```python
from build123d import *

# Parameters (mm, degrees)
F1_DEPTH = 27.813
F3_DEPTH = 6.3119
F5_DEPTH = 4.699
F7_DEPTH = 5.08


with BuildPart() as f1:
    # F0 (on Top) → F1 (new body)
    with BuildSketch(Plane.XY):
        with BuildLine():
            Line((-18.8019596104, 10.1706712406), (-18.8019596104, -14.8356287594))
            Line((-18.8019596104, -14.8356287594), (-12.4900596104, -14.8356287594))
            Line((-12.4900596104, -14.8356287594), (-12.4900596104, -1.8752787594))
            ThreePointArc((-12.4900596104, -1.8752787594), (-6.4067596104, 4.2080212406), (-0.3234596104, -1.8752787594))
            Line((-0.3234596104, -1.8752787594), (-0.3234596104, -14.8356287594))
            Line((-0.3234596104, -14.8356287594), (5.9884403896, -14.8356287594))
            Line((5.9884403896, -14.8356287594), (5.9884403896, 10.1706712406))
            Line((5.9884403896, 10.1706712406), (-18.8019596104, 10.1706712406))
        make_face()
    extrude(amount=F1_DEPTH)

    # F2 (on face) → F3 (cut, through all)
    with BuildSketch(Plane.YZ.offset(5.9884403896)):
        with BuildLine():
            ThreePointArc((-7.9141287594, 21.6408), (-8.4869693167, 23.0237594426), (-9.8699287594, 23.5966))
            Line((-9.8699287594, 23.5966), (-9.8699287594, 21.6408))
            Line((-9.8699287594, 21.6408), (-9.8699287594, 19.685))
            ThreePointArc((-9.8699287594, 19.685), (-8.4869693167, 20.2578405574), (-7.9141287594, 21.6408))
        make_face()
        with BuildLine():
            Line((-9.8699287594, 21.6408), (-9.8699287594, 23.5966))
            ThreePointArc((-9.8699287594, 23.5966), (-11.252888202, 23.0237594426), (-11.8257287594, 21.6408))
            Line((-11.8257287594, 21.6408), (-9.8699287594, 21.6408))
        make_face()
        with BuildLine():
            Line((-9.8699287594, 19.685), (-9.8699287594, 21.6408))
            Line((-9.8699287594, 21.6408), (-11.8257287594, 21.6408))
            ThreePointArc((-11.8257287594, 21.6408), (-11.252888202, 20.2578405574), (-9.8699287594, 19.685))
        make_face()
        with BuildLine():
            ThreePointArc((-7.8475873364, 5.3523653187), (-8.4441574212, 6.7586539368), (-9.8699287594, 7.3070330344))
            Line((-9.8699287594, 7.3070330344), (-9.8699287594, 5.4864))
            Line((-9.8699287594, 5.4864), (-9.8699287594, 3.3976976029))
            ThreePointArc((-9.8699287594, 3.3976976029), (-8.4441574212, 3.9460767006), (-7.8475873364, 5.3523653187))
        make_face()
        with BuildLine():
            Line((-9.8699287594, 5.4864), (-9.8699287594, 7.3070330344))
            ThreePointArc((-9.8699287594, 7.3070330344), (-11.1622464384, 6.7590122471), (-11.7545891057, 5.4864))
            Line((-11.7545891057, 5.4864), (-9.8699287594, 5.4864))
        make_face()
        with BuildLine():
            ThreePointArc((-11.7545891057, 5.4864), (-11.2554518403, 4.0421507116), (-9.8699287594, 3.3976976029))
            Line((-9.8699287594, 3.3976976029), (-9.8699287594, 5.4864))
            Line((-9.8699287594, 5.4864), (-11.7545891057, 5.4864))
        make_face()
    extrude(amount=-F3_DEPTH, mode=Mode.SUBTRACT)

    # F4 (on face) → F5 (join)
    with BuildSketch(Plane(origin=(0, 10.1706712406, 0), x_dir=(-1, 0, 0), z_dir=(0, 1, 0))):
        with BuildLine():
            ThreePointArc((-3.9818403896, 14.5669), (-1.9582997195, 9.6816406701), (2.9269596104, 7.6581))
            Line((2.9269596104, 7.6581), (2.9269596104, 13.34135))
            ThreePointArc((2.9269596104, 13.34135), (2.0603648947, 13.7003052843), (1.7014096104, 14.5669))
            Line((1.7014096104, 14.5669), (-3.9818403896, 14.5669))
        make_face()
        with BuildLine():
            Line((2.9269596104, 13.34135), (2.9269596104, 7.6581))
            ThreePointArc((2.9269596104, 7.6581), (7.8122189403, 9.6816406701), (9.8357596104, 14.5669))
            ThreePointArc((9.8357596104, 14.5669), (2.9269596104, 21.4757), (-3.9818403896, 14.5669))
            Line((-3.9818403896, 14.5669), (1.7014096104, 14.5669))
            ThreePointArc((1.7014096104, 14.5669), (2.0603648947, 15.4334947157), (2.9269596104, 15.79245))
            ThreePointArc((2.9269596104, 15.79245), (3.7935543261, 15.4334947157), (4.1525096104, 14.5669))
            ThreePointArc((4.1525096104, 14.5669), (3.7935543261, 13.7003052843), (2.9269596104, 13.34135))
        make_face()
    extrude(amount=F5_DEPTH)

    # F6 (on face) → F7 (cut)
    with BuildSketch(Plane(origin=(0, 10.1706712406, 0), x_dir=(-1, 0, 0), z_dir=(0, 1, 0))):
        with BuildLine():
            Line((3.5874825428, 23.4577979645), (6.1019596104, 27.813))
            Line((6.1019596104, 27.813), (-5.9884403896, 27.813))
            Line((-5.9884403896, 27.813), (-5.9884403896, 14.4474878907))
            Line((-5.9884403896, 14.4474878907), (-5.9881597655, 14.637636653))
            ThreePointArc((-5.9881597655, 14.637636653), (-3.11318956, 21.1244113541), (3.5874825428, 23.4577979645))
        make_face()
    extrude(amount=-F7_DEPTH, mode=Mode.SUBTRACT)


solid = f1.part
```
Work out the finished part from the listing and answer in its coordinate system (mm). A direction names the side the tool comes from. Round coordinates to 2 decimals unless told otherwise and drop trailing zeros. Loops run counter-clockwise (first coordinate to the right, second up) from the corner with the lowest first, then second, coordinate; pieces in that order, holes last. Notation, with made-up numbers: M 63.5,2.25 L 106.5,2.25 A10 cw 106.5,14.25 Z; hole C -29.5,33 d3. An arc over 180 degrees is marked long. One line per question, with ' | ' between items.
Q1. A tool of negligible diameter and unlimited length cuts with its end or side. For faces 1 (the flat face through (-12.49, -8, 14)), 2 (the flat face through (-12, 1, 27.813)), 3 (the flat face through (-3, 10.171, 15)), from which of +Z, -Z, +X, -X, +Y, -Y can it reach the whole face along a straight path? Write none if from no direction.
Conclusion:
face 1: +Z, -Z, -Y | face 2: +Z, +X, -X, +Y, -Y | face 3: +Y
Q2. Consider line 1 along X through (y, z) = (-3, 24.25); line 2 along Y through (x, z) = (4.5, 8); line 3 along Y through (x, z) = (0.5, 26.5). Determine where each line is inside the solid, lowest interval first. Write a range as from..to.
Conclusion:
line 1: x = -18.8..-12.49, -0.32..5.99 | line 2: y = -14.84..10.17 | line 3: y = -14.84..5.09
Q3. Find section D-D, the plane x = -5.5. Give the vertices of the cut face in (y, z), then the cut area to 3 significant figures.
Conclusion:
outline: M 4.14,0 L 10.17,0 L 10.17,8.16 L 14.87,8.16 L 14.87,20.98 L 10.17,20.98 L 10.17,26.77 L 5.09,26.77 L 5.09,27.81 L 4.14,27.81 Z | area: 223 mm2
Q4. Find section A-A, the plane y = -3. Give the vertices of the cut face in (x, z).
Conclusion:
outline: M -18.8,0 L -12.49,0 L -12.49,27.81 L -18.8,27.81 Z; M -0.32,0 L 5.99,0 L 5.99,27.81 L -0.32,27.81 Z
Q5. The mould has two halves that part along X. Classify faces 4 (the flat face through (-18.802, -2, 14)), 5 (the cylindrical face through (-6.541, 4.207, 13.712)), 6 (the flat face through (1, 5.091, 24)): +X half, -X half, draft (parallel to the pull), parting line (faces both ways), or undercut.
Conclusion:
face 4: -X half | face 5: undercut | face 6: draft
Q6. Find section C-C, the plane y = 12. Give the vertices of the cut face in (x, z).
Conclusion:
outline: C -2.93,14.57 d13.82; hole C -2.93,14.57 d2.45
Q7. Find section B-B, the plane z = 6. Give the vertices of the cut face in (x, y), then the cut area to 3 significant figures.
Conclusion:
outline: M -18.8,-14.84 L -12.49,-14.84 L -12.49,-1.88 A6.08 cw -0.32,-1.88 L -0.32,-7.96 L 5.99,-7.96 L 5.99,10.17 L -18.8,10.17 Z; M -0.32,-14.84 L 5.99,-14.84 L 5.99,-11.65 L -0.32,-11.65 Z | area: 381 mm2
Q8. Each of these flat-tipped pins is pushed along its axis until it touches: pin 1 Ø5 at (x, y) = (-12.5, 4) entering from -Z; pin 2 Ø1.5 at (x, z) = (-9, 8) entering from +Y. Where does it stop, or does it pass through?
Conclusion:
pin 1: stops at z = 0 | pin 2: stops at y = 10.17
